Work out the finished part from the listing and answer in its coordinate system (mm). A direction names the side the tool comes from. Give positions to 0.01 mm unless a question says otherwise; leave off trailing zeros. Write each loop counter-clockwise with the first axis right and the second up, starting at its lowest first coordinate (ties: lowest second). Pieces come first, ordered by that corner, then holes.
1) Find section A-A (x = 0). Determine the outline of the cut face in (y, z), plus the area to 3 significant figures.
2) A tool of negligible diameter and unlimited length cuts with its end or side. For faces 4 (the face through (10, 95, 12)), 5 (the face through (-3, 13, 25)), from which of +Z, -Z, +X, -X, +Y, -Y can it reach the whole face along a straight path? Write none if from no direction.
3) Determine the mould class of faces 1 (the face through (-10, 95, 12)), 2 (the face through (3, -82.924, 12)), 3 (the face through (-200, 11, 12)) for opening direction X: pulls with the +X half, pulls with the -X half, needs draft (parallel to the pull), parting line crosses it, or undercut.
4) A straight line is drawn through the part: probe 1 along X at (y, z) = (93, 23). Find the intervals that lie inside material, in ascending order.
Autodesk Inventor part; units mm, degrees
ref_plane "YZ Plane" through (0, 0, 0) normal (1, 0, 0) x (0, 1, 0)
ref_plane "XZ Plane" through (0, 0, 0) normal (0, 1, 0) x (-1, 0, 0)
ref_plane "XY Plane" through (0, 0, 0) normal (0, 0, 1) x (1, 0, 0)
sketch "Skizze1" plane through (0, 0, 0) normal (0, 0, 1) x (1, 0, 0)
  line L0 (-280, 0) -> (280, 0)
  line L1 (0, -126.7237) -> (0, 179.8763)
  line L2 (-200, 107.0763) -> (200, 107.0763)
  line L3 (200, 107.0763) -> (200, -82.9237)
  line L4 (200, -82.9237) -> (-200, -82.9237)
  line L5 (-200, -82.9237) -> (-200, 107.0763)
  point P0 (0, 0)
  dimension "d0" = 190
  dimension "d1" = 400
extrude "Extrusion1" add sketch "Skizze1" along normal blind 25
sketch "Skizze2" plane through (-200, 107.0763, 0) normal (0, 1, 0) x (1, 0, 0)
  line L0 (0, -25) -> (400, -25)
  point P0 (200, 0)
sketch "Skizze4" plane through (0, 0, 0) normal (0, 0, -1) x (-1, 0, 0)
  line L0 (-200, 107.0763) -> (200, 107.0763)
  line L1 (-10, 107.0763) -> (10, 107.0763)
  line L2 (10, 107.0763) -> (10, 83.161)
  line L3 (10, 83.161) -> (-10, 83.161)
  line L4 (-10, 83.161) -> (-10, 107.0763)
  circle A0 centre (0, 83.161) radius 10
  point P0 (0, 0)
  dimension "d12" = 20
  dimension "d13" = 10
extrude "Extrusion3" cut sketch "Skizze4" against normal blind 25
properties part number "Verkleidungsdeckel"
Results:
1. outline: (-82.92, 0) - (73.16, 0) - (73.16, 25) - (-82.92, 25) - close
1. area: 3,900 mm2
2. face 4: +Z, -Z, +Y
2. face 5: +Z, +X, -X, +Y, -Y
3. face 1: undercut
3. face 2: needs draft
3. face 3: pulls with the -X half
4. probe 1: x = -200 to -10, 10 to 200
